Input: part model. Units: mm. Frame: model coordinates. A direction names the side the tool comes from. Give positions to 0.01 mm unless a question says otherwise; leave off trailing zeros. Write each loop counter-clockwise with the first axis right and the second up, starting at its lowest first coordinate (ties: lowest second). Pieces come first, ordered by that corner, then holes. Notation, with made-up numbers: (8.5, 15) -> (29.5, 15) arc R30 ccw to (29.5, 44) -> close; hole circle Ø9 at (25, 31.5). An arc over 180 degrees is marked (long way). Return JSON: item names as keys, results as strings. Group by question number.
Item 1: Set-up query: faces 4 (the face through (2.09, -15, 1.25)), 5 (the face through (-54.836, -19.003, 1.252)), 6 (the face through (-50.8, 79, 4)), 7 (the face through (-41, 79, 2.54)), 8 (the face through (73, -63, 2.54)). Return all of +Z, -Z, +X, -X, +Y, -Y with unobstructed straight access to the full face (end or side cutting, diameter ignored); none if empty.
Item 2: Line query: line 1 (X direction, y = -5, z = 2.25); line 2 (X direction, y = -0.5, z = 6.25); line 3 (X direction, y = 32, z = 5). Output: solid intervals per line, ascending. Write a range as [from, to].
Item 3: Section C-C, the plane x = -42.5. Return loops of the section in (y, z).
Item 4: Section A-A, the plane z = 5.25. Return loops of the section in (x, y).
Item 5: Section B-B, the plane x = -8.5. Return loops of the section in (y, z), then the cut area to 3 significant figures.
Item 6: Mould query, pull axis Y, two halves, no side actions, for faces 1 (the face through (-39, -24, 6.35)), 2 (the face through (-22.47, 12.36, 1.25)), 3 (the face through (-58.444, -13.776, 1.252)). Classes: released by +Y, released by -Y, zero draft, split by the parting line, or undercut.
Item 7: Pin query (flat end, axial travel): P1, Ø11, axis at x = 28.5, y = -55.5, coming from the +Z side; P2, Ø3.5, axis at y = 81.5, z = 1.5, coming from the +X side; P3, Ø1.1, axis at x = -47, y = 79, coming from the -Z side; P4, Ø10, axis at x = -9.5, y = -7.5, coming from the -Z side. Return the tip coordinate at first contact, or that it passes through.
from build123d import *

# Parameters (mm, degrees)
F1_DEPTH = 6.35
F2_W     = 6.35
F2_H     = 50.8
F2_W_2   = 50.8
F2_H_2   = 6.35
F3_DEPTH = 2.54
F4_W     = 6.35
F4_H     = 6.35
F5_DEPTH = 6.35
F7_DEPTH = 3.81
F9_DEPTH = 3.81


with BuildPart() as f1:
    # F0 (on Top) → F1 (new body)
    with BuildSketch(Plane.XY):
        with BuildLine():
            Line((76.2, -82.55), (76.2, -76.2))
            ThreePointArc((76.2, -76.2), (-31.563073, -31.563073), (-76.2, 76.2))
            Line((-76.2, 76.2), (-82.55, 76.2))
            ThreePointArc((-82.55, 76.2), (-36.053202, -36.053202), (76.2, -82.55))
        make_face()
        with BuildLine():
            ThreePointArc((-50.8, 76.2), (-13.602561, -13.602561), (76.2, -50.8))
            Line((76.2, -50.8), (76.2, -44.45))
            ThreePointArc((76.2, -44.45), (-9.112433, -9.112433), (-44.45, 76.2))
            Line((-44.45, 76.2), (-50.8, 76.2))
        make_face()
    extrude(amount=F1_DEPTH)

    # F2 (on Top) → F3 (join)
    with BuildSketch(Plane.XY):
        with Locations((73.025, -63.5)):
            Rectangle(F2_W, F2_H)
        Polygon((25.181294, -80.819431), (40.879358, -32.50576), (34.840149, -30.543502), (19.142085, -78.857173), align=None)
        Polygon((-20.843345, -57.368706), (9.016146, -16.270642), (3.878888, -12.538206), (-25.980603, -53.636269), align=None)
        Polygon((-57.368706, -20.843345), (-16.270642, 9.016146), (-20.003079, 14.153404), (-61.101142, -15.706087), align=None)
        Polygon((-80.819431, 25.181294), (-32.50576, 40.879358), (-34.468018, 46.918566), (-82.781689, 31.220503), align=None)
        with Locations((-63.5, 79.375)):
            Rectangle(F2_W_2, F2_H_2)
    extrude(amount=F3_DEPTH)

    # F4 (on Top) → F5 (join)
    with BuildSketch(Plane.XY):
        with Locations((-79.375, 79.375)):
            Rectangle(F4_W, F4_H)
        with Locations((-47.625, 79.375)):
            Rectangle(F4_W, F4_H)
    extrude(amount=F5_DEPTH)

    # F6 (on face) → F7 (join)
    with BuildSketch(Plane(origin=(0, 0, 0), x_dir=(1, 0, 0), z_dir=(0, 0, -1))):
        with BuildLine():
            Line((76.2, 80.56626), (76.2, 79.37627))
            Line((76.2, 79.37627), (76.2, 78.18628))
            Line((76.2, 78.18628), (79.375, 78.18628))
            Line((79.375, 78.18628), (79.375, 77.47254))
            ThreePointArc((79.375, 77.47254), (81.210451, 79.37627), (79.375, 81.28))
            Line((79.375, 81.28), (79.375, 80.56626))
            Line((79.375, 80.56626), (76.2, 80.56626))
        make_face()
        with BuildLine():
            Line((76.2, 47.62373), (76.2, 46.43374))
            Line((76.2, 46.43374), (79.375, 46.43374))
            Line((79.375, 46.43374), (79.375, 45.72))
            ThreePointArc((79.375, 45.72), (81.210451, 47.62373), (79.375, 49.52746))
            Line((79.375, 49.52746), (79.375, 48.81372))
            Line((79.375, 48.81372), (76.2, 48.81372))
            Line((76.2, 48.81372), (76.2, 47.62373))
        make_face()
    extrude(amount=-F7_DEPTH)

    # F8 (on face) → F9 (cut)
    with BuildSketch(Plane(origin=(0, 0, 0), x_dir=(1, 0, 0), z_dir=(0, 0, -1))):
        with BuildLine():
            Line((-80.56626, -82.55), (-79.37627, -82.55))
            Line((-79.37627, -82.55), (-78.18628, -82.55))
            Line((-78.18628, -82.55), (-78.18628, -79.375))
            Line((-78.18628, -79.375), (-77.47254, -79.375))
            ThreePointArc((-77.47254, -79.375), (-79.37627, -77.539549), (-81.28, -79.375))
            Line((-81.28, -79.375), (-80.56626, -79.375))
            Line((-80.56626, -79.375), (-80.56626, -82.55))
        make_face()
        with BuildLine():
            Line((-49.52746, -79.375), (-48.81372, -79.375))
            Line((-48.81372, -79.375), (-48.81372, -82.55))
            Line((-48.81372, -82.55), (-47.62373, -82.55))
            Line((-47.62373, -82.55), (-46.43374, -82.55))
            Line((-46.43374, -82.55), (-46.43374, -79.375))
            Line((-46.43374, -79.375), (-45.72, -79.375))
            ThreePointArc((-45.72, -79.375), (-47.62373, -77.539549), (-49.52746, -79.375))
        make_face()
    extrude(amount=-F9_DEPTH, mode=Mode.SUBTRACT)


solid = f1.part
Answer below:
{
 "1": {"face 4": "+Z, -Z, +Y", "face 5": "+Z, -Z, -Y", "face 6": "+Z, +Y", "face 7": "+Z, +X, +Y", "face 8": "+Z, +X"},
 "2": {"line 1": "x = [-60.21, -52.77], [-46.37, -35.56], [-21.45, -13.04]", "line 2": "x = [-62.79, -55.49], [-25.02, -16.93]", "line 3": "x = [-76.27, -69.65], [-42.86, -36.06]"},
 "3": {"outline": "(-29.21, 0) -> (-19.38, 0) -> (-19.38, 6.35) -> (-29.21, 6.35) -> close; (-10.04, 0) -> (-2.19, 0) -> (-2.19, 2.54) -> (-10.04, 2.54) -> close; (31.04, 0) -> (54.6, 0) -> (54.6, 6.35) -> (31.04, 6.35) -> close; (76.2, 0) -> (82.55, 0) -> (82.55, 2.54) -> (76.2, 2.54) -> close"},
 "4": {"outline": "(-82.55, 76.2) arc R158.75 ccw to (76.2, -82.55) -> (76.2, -76.2) arc R152.4 cw to (-76.2, 76.2) -> (-76.2, 82.55) -> (-82.55, 82.55) -> close; (-50.8, 76.2) arc R127 ccw to (76.2, -50.8) -> (76.2, -44.45) arc R120.65 cw to (-44.45, 76.2) -> (-44.45, 82.55) -> (-50.8, 82.55) -> close"},
 "5": {"outline": "(-58.07, 0) -> (-50.5, 0) -> (-50.5, 6.35) -> (-58.07, 6.35) -> close; (-40.38, 0) -> (-29.58, 0) -> (-29.58, 2.54) -> (-40.38, 2.54) -> close; (-18.43, 0) -> (-9.72, 0) -> (-9.72, 6.35) -> (-18.43, 6.35) -> close", "area": "131 mm2"},
 "6": {"face 1": "zero draft", "face 2": "released by +Y", "face 3": "undercut"},
 "7": {"P1": "stops at z = 2.54", "P2": "stops at x = -38.1", "P3": "stops at z = 3.81", "P4": "stops at z = 0"}
}
